Geometry check sheet. Reference: the model listing, model coordinates, mm. Give positions to 0.01 mm unless a question says otherwise; leave off trailing zeros. Loops run counter-clockwise (first coordinate to the right, second up) from the corner with the lowest first, then second, coordinate; pieces in that order, holes last. Notation, with made-up numbers: (55, -21.5) -> (74, -21.5) arc R20 ccw to (74, -1.5) -> close; hole circle Ø1 at (49.25, -3.5). An arc over 180 degrees is marked (long way). Write each question's results on one line, items separated by ' | '. Start each with the question number.
1) Sectioned sample at A-A on x = 0. Record the cut outline in (y, z), then the cut area to 3 significant figures.
2) Depth check by flat-ended pin: pin 1 (1.5 mm diameter, centred on x = -98.5, z = 1, fed in from -Y); pin 2 (0.9 mm diameter, centred on x = 79, z = 1, fed in from +Y); pin 3 (1 mm diameter, centred on y = -24, z = 2, fed in from -X). Enter the tip coordinate at first touch or a pass-through.
3) Sectioned sample at C-C on z = 0.5. Count the separate pieces of the cut face and the enclosed holes in it, then the cut area to 3 significant figures.
4) Draft check along X on faces 1 (the face through (-76.6, 0.26, 1.52)), 2 (the face through (-1, 0, 3)). Enter one of: pulls with the +X half, pulls with the -X half, needs draft (parallel to the pull), parting line crosses it, or undercut.
5) Sectioned sample at B-B on y = 0. Record the cut outline in (x, z), then the cut area to 3 significant figures.
6) Scan lines: line 1 (X direction, y = -18, z = 1.7); line 2 (X direction, y = -15, z = 1.95); line 3 (Y direction, x = 0, z = 1). Record each from-to range of solid material in increasing order. Write a range as from..to.
```python
from build123d import *

# Parameters (mm, degrees)
SALIENTE_EXTRUIR2_DEPTH = 3
CROQUIS3_R              = 5.85
CORTAR_EXTRUIR1_DEPTH   = 3
CROQUIS4_W              = 13
CROQUIS4_H              = 8.6
CORTAR_EXTRUIR2_DEPTH   = 3
CROQUIS5_R              = 5.8
CORTAR_EXTRUIR3_DEPTH   = 3


with BuildPart() as part:
    # Croquis1 → Saliente-Extruir2 (new body)
    with BuildSketch(Plane.XY):
        Polygon((-71.428571429, -31.9), (-71.428571429, -35), (-42.857142857, -35), (-42.857142857, -31.9), (-14.285714286, -31.9), (-14.285714286, -35), (14.285714286, -35), (14.285714286, -31.9), (42.857142857, -31.9), (42.857142857, -35), (71.428571429, -35), (71.428571429, -31.9), (96.9, -31.9), (96.9, -21), (100, -21), (100, -7), (96.9, -7), (96.9, 7), (100, 7), (100, 21), (96.9, 21), (96.9, 31.9), (71.428571429, 31.9), (71.428571429, 35), (42.857142857, 35), (42.857142857, 31.9), (14.285714286, 31.9), (14.285714286, 35), (-14.285714286, 35), (-14.285714286, 31.9), (-42.857142857, 31.9), (-42.857142857, 35), (-71.428571429, 35), (-71.428571429, 31.9), (-96.9, 31.9), (-96.9, 21), (-100, 21), (-100, 7), (-96.9, 7), (-96.9, -7), (-100, -7), (-100, -21), (-96.9, -21), (-96.9, -31.9), align=None)
    extrude(amount=SALIENTE_EXTRUIR2_DEPTH)

    # Croquis3 → Cortar-Extruir1 (cut)
    with BuildSketch(Plane.XY.offset(3)):
        with Locations((-70.755124627, 0)):
            Circle(CROQUIS3_R)
    extrude(amount=-CORTAR_EXTRUIR1_DEPTH, mode=Mode.SUBTRACT)

    # Croquis4 → Cortar-Extruir2 (cut)
    with BuildSketch(Plane.XY.offset(3)):
        with Locations((65.03625281, -15.995927208)):
            Rectangle(CROQUIS4_W, CROQUIS4_H)
    extrude(amount=-CORTAR_EXTRUIR2_DEPTH, mode=Mode.SUBTRACT)

    # Croquis5 → Cortar-Extruir3 (cut)
    with BuildSketch(Plane(origin=(0, 0, 0), x_dir=(-1, 0, 0), z_dir=(0, 0, -1))):
        with Locations((0, -15.950666175)):
            Circle(CROQUIS5_R)
    extrude(amount=-CORTAR_EXTRUIR3_DEPTH, mode=Mode.SUBTRACT)


solid = part.part
```
Result:
1) outline: (-35, 0) -> (-21.75, 0) -> (-21.75, 3) -> (-35, 3) -> close; (-10.15, 0) -> (35, 0) -> (35, 3) -> (-10.15, 3) -> close | area: 175 mm^2
2) pin 1: y = -21 | pin 2: y = 31.9 | pin 3: x = -96.9
3) separate pieces: 1 | enclosed holes: 3 | area: 12,700 mm^2
4) face 1: undercut | face 2: needs draft
5) outline: (-96.9, 0) -> (-76.61, 0) -> (-76.61, 3) -> (-96.9, 3) -> close; (-64.91, 0) -> (96.9, 0) -> (96.9, 3) -> (-64.91, 3) -> close | area: 546 mm^2
6) line 1: -100..-5.43, 5.43..58.54, 71.54..100 | line 2: -100..-5.72, 5.72..58.54, 71.54..100 | line 3: -35..-21.75, -10.15..35
